Geometry check sheet. Reference: the model listing, model coordinates, mm. A direction names the side the tool comes from. Round coordinates to 2 decimals unless told otherwise and drop trailing zeros. Write each loop counter-clockwise with the first axis right and the second up, starting at its lowest first coordinate (ties: lowest second). Pieces come first, ordered by that corner, then holes. Notation, with made-up numbers: (-31, -26) -> (10, -26) arc R11 cw to (10, -21) -> close; hole circle Ø4 at (16.5, 47.5). An arc over 180 degrees is marked (long way). Use a Markdown table: item, result.
```python
from build123d import *

# Parameters (mm, degrees)
SKETCH1_R            = 12.5
BOSS_EXTRUDE1_DEPTH  = 10
FILLET1_R            = 5
SKETCH1_2_R          = 12.5
BOSS_EXTRUDE2_DEPTH  = 30
SKETCH2_R            = 12.5
BOSS_EXTRUDE3_DEPTH  = 50
FILLET1_OF_MIRROR1_R = 5


with BuildPart() as part:
    # Sketch1 → Boss-Extrude1 (new body)
    with BuildSketch(Plane.XY):
        with BuildLine():
            Line((-50, 0), (-23.941410033, 0))
            Line((-23.941410033, 0), (-17.234135678, 38.038843109))
            ThreePointArc((-17.234135678, 38.038843109), (0, 52.5), (17.234135678, 38.038843109))
            Line((17.234135678, 38.038843109), (23.941410033, 0))
            Line((23.941410033, 0), (50, 0))
            ThreePointArc((50, 0), (0, -50), (-50, 0))
        make_face()
        Circle(SKETCH1_R, mode=Mode.SUBTRACT)
    boss_extrude1 = extrude(amount=BOSS_EXTRUDE1_DEPTH)

    # Fillet1
    fillet1_edges = [part.edges().sort_by_distance(p)[0] for p in [
        (-50, 0, 5),
        (-23.941410033, 0, 5),
        (23.941410033, 0, 5),
        (50, 0, 5),
    ]]
    fillet(fillet1_edges, radius=FILLET1_R)

    # Sketch1<2> → Boss-Extrude2 (add)
    with BuildSketch(Plane.XY):
        Circle(SKETCH1_2_R)
    boss_extrude2 = extrude(amount=BOSS_EXTRUDE2_DEPTH)

    # Sketch2 → Boss-Extrude3 (add)
    with BuildSketch(Plane(origin=(0, 0, 0), x_dir=(-1, 0, 0), z_dir=(0, 0, -1))):
        with Locations((0, 35)):
            Circle(SKETCH2_R)
    extrude(amount=BOSS_EXTRUDE3_DEPTH)

    # Mirror1: Boss-Extrude1, Boss-Extrude2 across plane
    add(boss_extrude1.mirror(Plane(origin=(0, 0, -25), x_dir=(1, 0, 0), z_dir=(0, 0, -1))))
    add(boss_extrude2.mirror(Plane(origin=(0, 0, -25), x_dir=(1, 0, 0), z_dir=(0, 0, -1))))

    # Fillet1 of Mirror1
    fillet1_of_mirror1_edges = [part.edges().sort_by_distance(p)[0] for p in [
        (-50, 0, -55),
        (-23.941410033, 0, -55),
        (23.941410033, 0, -55),
        (50, 0, -55),
    ]]
    fillet(fillet1_of_mirror1_edges, radius=FILLET1_OF_MIRROR1_R)


solid = part.part
```
(1) Gauge pin test, flat ends, axial feed: pin 1 Ø3 at (y, z) = (2, 13) entering from -X; pin 2 Ø12 at (x, z) = (-39, 10) entering from -Y; pin 3 Ø12 at (x, y) = (29.5, -7) entering from +Z; pin 4 Ø6 at (x, z) = (36.5, -44.5) entering from +Y. Record the tip position at first contact, or that the pin passes through.
A:
| item | result |
|---|---|
| pin 1 | stops at x = -12.49 |
| pin 2 | stops at y = -37.56 |
| pin 3 | stops at z = 10 |
| pin 4 | passes through |
(2) Section check C-C on x = -4.5. Record the cut outline in (y, z), plus the area to 3 significant figures.
A:
| item | result |
|---|---|
| outline | (-49.8, -60) -> (-11.66, -60) -> (-11.66, -80) -> (11.66, -80) -> (11.66, -60) -> (51.91, -60) -> (51.91, -50) -> (46.66, -50) -> (46.66, 0) -> (51.91, 0) -> (51.91, 10) -> (11.66, 10) -> (11.66, 30) -> (-11.66, 30) -> (-11.66, 10) -> (-49.8, 10) -> (-49.8, 0) -> (23.34, 0) -> (23.34, -50) -> (-49.8, -50) -> close |
| area | 4,130 mm2 |
(3) Section check D-D on z = -27.5. Record the cut outline in (x, y).
A:
| item | result |
|---|---|
| outline | circle Ø25 at (0, 35) |
(4) Section check B-B on x = 15. Record the cut outline in (y, z), plus the area to 3 significant figures.
A:
| item | result |
|---|---|
| outline | (-47.7, -60) -> (44.01, -60) -> (44.01, -50) -> (-47.7, -50) -> close; (-47.7, 0) -> (44.01, 0) -> (44.01, 10) -> (-47.7, 10) -> close |
| area | 1,830 mm2 |
(5) Release check for a two-part mould opening along Z. For faces 1 (the face through (-0.342, 52.497, -54.93)), 2 (the face through (0, 0, -80)), 3 (the face through (1, -9, -50)) record: +Z half, -Z half, draft (parallel to the pull), parting line (faces both ways), or undercut.
A:
| item | result |
|---|---|
| face 1 | draft |
| face 2 | -Z half |
| face 3 | undercut |
(6) Section check A-A on y = 20. Record the cut outline in (x, z).
A:
| item | result |
|---|---|
| outline | (-20.41, -60) -> (20.41, -60) -> (20.41, -50) -> (-20.41, -50) -> close; (-20.41, 0) -> (20.41, 0) -> (20.41, 10) -> (-20.41, 10) -> close |
(7) Thickness scan on line 1 (Z direction, x = 17.5, y = 11); line 2 (Y direction, x = 0.5, z = -74); line 3 (X direction, y = -5, z = -68). Record the ranges inside material, lowest first.
A:
| item | result |
|---|---|
| line 1 | z = -60 to -50, 0 to 10 |
| line 2 | y = -12.49 to 12.49 |
| line 3 | x = -11.46 to 11.46 |
(8) Access from +Z, -Z, +X, -X, +Y, -Y to the whole of each face (thin tool, end or side, straight path). Record for faces 4 (the face through (2.71, 22.797, -24.65)), 5 (the face through (36, 0, 5)), 6 (the face through (-37, 0, 5)), 7 (the face through (11.923, 3.755, -69.86)).
A:
| item | result |
|---|---|
| face 4 | none |
| face 5 | +Z, -Z, +X, +Y |
| face 6 | +Z, -Z, -X, +Y |
| face 7 | -Z |
